Verification items for the finished model (mm, model axes). A direction names the side the tool comes from. Round coordinates to 2 decimals unless told otherwise and drop trailing zeros. Loops run counter-clockwise (first coordinate to the right, second up) from the corner with the lowest first, then second, coordinate; pieces in that order, holes last. Notation, with made-up numbers: M 38,41.25 L 71,41.25 A22 cw 71,72.25 Z; hole C 35,73.5 d6. An arc over 180 degrees is marked long. One line per item, written item: value.
from build123d import *

# Parameters (mm, degrees)
SKETCH_1_W          = 61
SKETCH_1_H          = 4
EXTRUDE_1_DEPTH     = 15
EXTRUDE_1_2_DEPTH   = 15
SKETCH_2_W          = 61
SKETCH_2_H          = 23
EXTRUDE_2_DEPTH     = 4
EXTRUDE_3_DEPTH     = 23
CUT_EXTRUDE_1_DEPTH = 23
CUT_EXTRUDE_2_DEPTH = 23
CUT_EXTRUDE_3_DEPTH = 23
FILLET_1_R          = 1
SKETCH_9_W          = 2
SKETCH_9_H          = 16
CUT_EXTRUDE_4_DEPTH = 40
FILLET_2_R          = 1
SKETCH_10_W         = 25.473517425
SKETCH_10_H         = 15
CUT_EXTRUDE_5_DEPTH = 40
FILLET_3_R          = 1
EXTRUDE_4_DEPTH     = 4
CUT_EXTRUDE_6_DEPTH = 40


with BuildPart() as part:
    # Sketch 1 → Extrude 1 (new body)
    with BuildSketch(Plane(origin=(0, 0, 0), x_dir=(1, 0, 0), z_dir=(0, 1, 0))):
        with Locations((-29.49872666, -14.866833958)):
            Rectangle(SKETCH_1_W, SKETCH_1_H)
    extrude(amount=EXTRUDE_1_DEPTH)



with BuildPart() as body_2:
    # Sketch 1 → Extrude 1 2 (new body)
    with BuildSketch(Plane(origin=(0, 0, 0), x_dir=(1, 0, 0), z_dir=(0, 1, 0))):
        with Locations((-29.49872666, -33.866833958)):
            Rectangle(SKETCH_1_W, SKETCH_1_H)
    extrude(amount=EXTRUDE_1_2_DEPTH)


with BuildPart() as part_1:
    add(part.part)

    add(body_2.part)  # Extrude 2 merges body 2
    # Sketch 2 → Extrude 2 (add)
    with BuildSketch(Plane(origin=(0, 15, 0), x_dir=(1, 0, 0), z_dir=(0, 1, 0))):
        with Locations((-29.49872666, -24.366833958)):
            Rectangle(SKETCH_2_W, SKETCH_2_H)
    extrude(amount=EXTRUDE_2_DEPTH)

    # Sketch 3 → Extrude 3 (add)
    with BuildSketch(Plane.XY.offset(35.866833958)):
        with BuildLine():
            Line((-59.99872666, 25), (-59.99872666, 19))
            Line((-59.99872666, 19), (-45.633143428, 19))
            ThreePointArc((-45.633143428, 19), (-53.008133433, 21.539826341), (-59.99872666, 25))
        make_face()
        with BuildLine():
            ThreePointArc((1.00127334, 25), (-5.989319887, 21.539826341), (-13.364309893, 19))
            Line((-13.364309893, 19), (1.00127334, 19))
            Line((1.00127334, 19), (1.00127334, 25))
        make_face()
    extrude(amount=-EXTRUDE_3_DEPTH)

    # Sketch 4 → Cut-Extrude 1 (cut)
    with BuildSketch(Plane.XY.offset(35.866833958)):
        with BuildLine():
            Line((-59.99872666, 25), (1.00127334, 25))
            ThreePointArc((1.00127334, 25), (-29.49872666, 16.827549631), (-59.99872666, 25))
        make_face()
    extrude(amount=-CUT_EXTRUDE_1_DEPTH, mode=Mode.SUBTRACT)

    # Sketch 7 → Cut-Extrude 2 (cut)
    with BuildSketch(Plane.XY.offset(35.866833958)):
        with BuildLine():
            Line((-44.49872666, 0), (-29.49872666, 0))
            Line((-29.49872666, 0), (-29.49872666, 14))
            ThreePointArc((-29.49872666, 14), (-35.843538639, 14.163021123), (-42.13706744, 14.984428559))
            ThreePointArc((-42.13706744, 14.984428559), (-43.778703527, 14.554168766), (-44.49872666, 13.017399681))
            Line((-44.49872666, 13.017399681), (-44.49872666, 0))
        make_face()
        with BuildLine():
            Line((-54.49872666, 0), (-54.49872666, 17.322648745))
            ThreePointArc((-54.49872666, 17.322648745), (-54.823583781, 18.41530438), (-55.692622995, 19.15300305))
            ThreePointArc((-55.692622995, 19.15300305), (-57.866323827, 20.161752214), (-59.99872666, 21.255099523))
            Line((-59.99872666, 21.255099523), (-59.99872666, 0))
            Line((-59.99872666, 0), (-54.49872666, 0))
        make_face()
    cut_extrude_2 = extrude(amount=-CUT_EXTRUDE_2_DEPTH, mode=Mode.SUBTRACT)

    # Sketch 8 → Cut-Extrude 3 (cut)
    with BuildSketch(Plane.XY.offset(35.866833958)):
        with BuildLine():
            Line((-59.99872666, 24), (-59.99872666, 25))
            Line((-59.99872666, 25), (-52.99872666, 25))
            Line((-52.99872666, 25), (-52.99872666, 20.59639466))
            ThreePointArc((-52.99872666, 20.59639466), (-56.552305579, 22.188004639), (-59.99872666, 24))
        make_face()
    cut_extrude_3 = extrude(amount=-CUT_EXTRUDE_3_DEPTH, mode=Mode.SUBTRACT)

    # Fillet 1
    fillet_1_edges = [part_1.edges().sort_by_distance(p)[0] for p in [
        (-59.99872666, 21.255099523, 24.366833958),
        (-59.99872666, 24, 24.366833958),
    ]]
    fillet(fillet_1_edges, radius=FILLET_1_R)

    # Sketch 9 → Cut-Extrude 4 (cut)
    with BuildSketch(Plane.XZ):
        with Locations((-55.49872666, 24.366833958)):
            Rectangle(SKETCH_9_W, SKETCH_9_H)
    cut_extrude_4 = extrude(amount=-CUT_EXTRUDE_4_DEPTH, mode=Mode.SUBTRACT)

    # Mirror 3: Cut-Extrude 2 across plane
    add(cut_extrude_2.mirror(Plane.ZY.offset(29.49872666)), mode=Mode.SUBTRACT)

    # Mirror 4: Cut-Extrude 3 across plane
    add(cut_extrude_3.mirror(Plane.ZY.offset(29.49872666)), mode=Mode.SUBTRACT)

    # Fillet 2
    fillet_2_edges = [part_1.edges().sort_by_distance(p)[0] for p in [
        (1.00127334, 21.255099523, 24.366833958),
        (1.00127334, 24, 24.366833958),
    ]]
    fillet(fillet_2_edges, radius=FILLET_2_R)

    # Mirror 7: Cut-Extrude 4 across plane
    add(cut_extrude_4.mirror(Plane.ZY.offset(29.49872666)), mode=Mode.SUBTRACT)

    # Sketch 10 → Cut-Extrude 5 (cut)
    with BuildSketch(Plane.XZ):
        with Locations((-29.498726661, 24.366833958)):
            Rectangle(SKETCH_10_W, SKETCH_10_H)
    extrude(amount=-CUT_EXTRUDE_5_DEPTH, mode=Mode.SUBTRACT)

    # Fillet 3
    fillet_3_edges = [part_1.edges().sort_by_distance(p)[0] for p in [
        (-16.761967948, 16.586040333, 16.866833958),
        (-42.235485373, 16.586040333, 16.866833958),
        (-42.235485373, 16.586040333, 31.866833958),
        (-16.761967948, 16.586040333, 31.866833958),
    ]]
    fillet(fillet_3_edges, radius=FILLET_3_R)

    # Sketch 11 → Extrude 4 (add)
    with BuildSketch(Plane.XY.offset(35.866833958)):
        with BuildLine():
            Line((-52.99872666, 21.535898385), (-38.761178229, 25.332577966))
            ThreePointArc((-38.761178229, 25.332577966), (-38.087895944, 25.656566573), (-37.580506922, 26.205049966))
            Line((-37.580506922, 26.205049966), (-33.586227985, 32.595896265))
            ThreePointArc((-33.586227985, 32.595896265), (-32.859768442, 33.285183347), (-31.890231377, 33.535898385))
            Line((-31.890231377, 33.535898385), (-27.107221943, 33.535898385))
            ThreePointArc((-27.107221943, 33.535898385), (-26.137684878, 33.285183347), (-25.411225335, 32.595896265))
            Line((-25.411225335, 32.595896265), (-21.416946398, 26.205049966))
            ThreePointArc((-21.416946398, 26.205049966), (-20.909557376, 25.656566573), (-20.236275091, 25.332577966))
            Line((-20.236275091, 25.332577966), (-5.99872666, 21.535898385))
            ThreePointArc((-5.99872666, 21.535898385), (-29.49872666, 16.827549631), (-52.99872666, 21.535898385))
        make_face()
    extrude(amount=-EXTRUDE_4_DEPTH)

    # Sketch 13 → Cut-Extrude 6 (cut)
    with BuildSketch(Plane.XY.offset(35.866833958)):
        with BuildLine():
            Line((-31.629734398, 30.065897325), (-35.591020119, 23.727840171))
            ThreePointArc((-35.591020119, 23.727840171), (-35.725277784, 23.010296005), (-35.336096399, 22.392693705))
            Line((-35.336096399, 22.392693705), (-30.091801244, 18.529726902))
            ThreePointArc((-30.091801244, 18.529726902), (-29.49872666, 18.334874428), (-28.905652077, 18.529726902))
            Line((-28.905652077, 18.529726902), (-23.661356922, 22.392693705))
            ThreePointArc((-23.661356922, 22.392693705), (-23.272175536, 23.010296005), (-23.406433201, 23.727840171))
            Line((-23.406433201, 23.727840171), (-27.367718922, 30.065897325))
            ThreePointArc((-27.367718922, 30.065897325), (-27.730948694, 30.410540866), (-28.215717226, 30.535898385))
            Line((-28.215717226, 30.535898385), (-30.781736094, 30.535898385))
            ThreePointArc((-30.781736094, 30.535898385), (-31.266504627, 30.410540866), (-31.629734398, 30.065897325))
        make_face()
        with BuildLine():
            Line((-39.022032341, 22.158181931), (-46.415604198, 20.186562769))
            ThreePointArc((-46.415604198, 20.186562769), (-46.786746411, 19.708589315), (-46.425517056, 19.2230808))
            ThreePointArc((-46.425517056, 19.2230808), (-39.690366454, 17.684965064), (-32.824491011, 16.918278649))
            ThreePointArc((-32.824491011, 16.918278649), (-32.326643896, 17.248573111), (-32.500693355, 17.820108732))
            Line((-32.500693355, 17.820108732), (-38.171295107, 21.997094517))
            ThreePointArc((-38.171295107, 21.997094517), (-38.578325126, 22.174488298), (-39.022032341, 22.158181931))
        make_face()
        with BuildLine():
            Line((-19.97542098, 22.158181931), (-12.581849122, 20.186562769))
            ThreePointArc((-12.581849122, 20.186562769), (-12.210706909, 19.708589315), (-12.571936264, 19.2230808))
            ThreePointArc((-12.571936264, 19.2230808), (-19.307086867, 17.684965064), (-26.17296231, 16.918278649))
            ThreePointArc((-26.17296231, 16.918278649), (-26.670809424, 17.248573111), (-26.496759965, 17.820108732))
            Line((-26.496759965, 17.820108732), (-20.826158214, 21.997094517))
            ThreePointArc((-20.826158214, 21.997094517), (-20.419128195, 22.174488298), (-19.97542098, 22.158181931))
        make_face()
    extrude(amount=-CUT_EXTRUDE_6_DEPTH, mode=Mode.SUBTRACT)


solid = part_1.part
(1) Thickness scan on L1, parallel to X at y = 17, z = 23.75; L2, parallel to X at y = 3, z = 34.5; L3, parallel to X at y = 16, z = 33.25. Record the ranges inside material, lowest first. Write a range as from..to.
Completed:
L1: x = -54.5..-42.24, -16.76..-4.5
L2: x = -54.5..-44.5, -14.5..-4.5
L3: x = -54.5..-4.5
(2) Sectioned sample at A-A on z = 22.5. Enter the section's corners in (x, y), and give its area (3 significant figures).
Completed:
outline: M -60,21.86 A1 ccw -59.46,20.97 A61 ccw -56.5,19.52 L -56.5,22.16 A61.87 cw -58.53,23.19 A1 ccw -60,22.31 Z; M -54.5,15 L -42.76,15 A2 cw -42.24,15 L -42.24,18.17 A61 cw -53,21.54 L -53,20.6 A61.87 cw -54.5,21.24 Z; M -16.76,15 A2 cw -16.24,15 L -4.5,15 L -4.5,21.24 A61.87 cw -6,20.6 L -6,21.54 A61 cw -16.76,18.17 Z; M -2.5,19.52 A61 ccw 0.47,20.97 A1 ccw 1,21.86 L 1,22.31 A1 ccw -0.47,23.19 A61.87 cw -2.5,22.16 Z
area: 136 mm^2
(3) Mould release check, pull along Z, two halves, no side actions. Record for faces 1 (the face through (-42.235, 17, 24)), 2 (the face through (-50, 0, 34)): +Z half, -Z half, draft (parallel to the pull), parting line (faces both ways), or undercut.
Completed:
face 1: undercut
face 2: draft
(4) Sectioned sample at D-D on z = 15.25. Enter the section's corners in (x, y).
Completed:
outline: M -60,21.86 A1 ccw -59.46,20.97 A61 ccw -55.69,19.15 A2 cw -54.5,17.32 L -54.5,0 L -44.5,0 L -44.5,13.02 A2 cw -42.14,14.98 A61 ccw -29.5,14 A61 ccw -16.86,14.98 A2 cw -14.5,13.02 L -14.5,0 L -4.5,0 L -4.5,17.32 A2 cw -3.3,19.15 A61 ccw 0.47,20.97 A1 ccw 1,21.86 L 1,22.31 A1 ccw -0.47,23.19 A61.87 cw -6,20.6 L -6,21.54 A61 cw -53,21.54 L -53,20.6 A61.87 cw -58.53,23.19 A1 ccw -60,22.31 Z
(5) Sectioned sample at C-C on y = 29. Enter the section's corners in (x, z), and give its area (3 significant figures).
Completed:
outline: M -35.83,31.87 L -32.3,31.87 L -32.3,35.87 L -35.83,35.87 Z; M -26.7,31.87 L -23.16,31.87 L -23.16,35.87 L -26.7,35.87 Z
area: 28.3 mm^2
(6) Tool access check on faces 3 (the face through (-45.98, 23.408, 33.895)), 4 (the face through (-2.499, 21, 24)), 5 (the face through (-14.499, 7, 15)), 6 (the face through (-23.274, 23, 33.895)). Record the directions out of +Z, -Z, +X, -X, +Y, -Y that give a thin tool (end or side, any length) a straight path to the whole face; none if there is none.
Completed:
face 3: +Z, -Z, +Y
face 4: +Y, -Y
face 5: +Z, -Z, -Y
face 6: +Z, -Z
(7) Depth check by flat-ended pin: pin 1 Ø1 at (x, z) = (-49.5, 15.5) entering from +Y; pin 2 Ø1.5 at (x, z) = (-53, 29) entering from -Y; pin 3 Ø1.2 at (y, z) = (4, 34) entering from +X. Enter the tip coordinate at first touch or a pass-through.
Completed:
pin 1: stops at y = 20.38
pin 2: stops at y = 15
pin 3: stops at x = -4.5
(8) Sectioned sample at B-B on y = 9. Enter the section's corners in (x, z).
Completed:
outline: M -54.5,12.87 L -44.5,12.87 L -44.5,16.87 L -54.5,16.87 Z; M -54.5,31.87 L -44.5,31.87 L -44.5,35.87 L -54.5,35.87 Z; M -14.5,12.87 L -4.5,12.87 L -4.5,16.87 L -14.5,16.87 Z; M -14.5,31.87 L -4.5,31.87 L -4.5,35.87 L -14.5,35.87 Z
